```python
from build123d import *

# Parameters (mm, degrees)
PCB_START                  = -40
SK_PCB_W                   = 85
SK_PCB_H                   = 56
PCB_DEPTH                  = 1.6
BARRENOS_M2_5_START        = -40
SK_BARRENOS_M2_5_R         = 1.35
BARRENOS_M2_5_DEPTH        = 1.6
ETHERNET_START             = -38.4
SK_ETHERNET_W              = 21
SK_ETHERNET_H              = 16
ETHERNET_DEPTH             = 13.5
USB_START                  = -38.4
SK_USB_W                   = 17.5
SK_USB_H                   = 13
USB_DEPTH                  = 16
DISIPADOR_VENTILADOR_START = -38.4
SK_DISIPADOR_VENTILADOR_W  = 40
SK_DISIPADOR_VENTILADOR_H  = 38
DISIPADOR_VENTILADOR_DEPTH = 10


with BuildPart() as part:
    # Sk_PCB → PCB (new body)
    with BuildSketch(Plane.XY.offset(PCB_START)):
        with Locations((-52.5, 0)):
            Rectangle(SK_PCB_W, SK_PCB_H)
    extrude(amount=PCB_DEPTH)

    # Sk_Barrenos_M2-5 → Barrenos_M2-5 (cut)
    with BuildSketch(Plane.XY.offset(BARRENOS_M2_5_START)):
        with Locations((-13.5, -24.5)):
            Circle(SK_BARRENOS_M2_5_R)
        with Locations((-13.5, 24.5)):
            Circle(SK_BARRENOS_M2_5_R)
        with Locations((-71.5, -24.5)):
            Circle(SK_BARRENOS_M2_5_R)
        with Locations((-71.5, 24.5)):
            Circle(SK_BARRENOS_M2_5_R)
    extrude(amount=BARRENOS_M2_5_DEPTH, mode=Mode.SUBTRACT)

    # Sk_Ethernet → Ethernet (add)
    with BuildSketch(Plane.XY.offset(ETHERNET_START)):
        with Locations((-87.5, 16)):
            Rectangle(SK_ETHERNET_W, SK_ETHERNET_H)
    extrude(amount=ETHERNET_DEPTH)

    # Sk_USB → USB (add)
    with BuildSketch(Plane.XY.offset(USB_START)):
        with Locations((-89.25, -19.5)):
            Rectangle(SK_USB_W, SK_USB_H)
        with Locations((-89.25, -3.5)):
            Rectangle(SK_USB_W, SK_USB_H)
    extrude(amount=USB_DEPTH)

    # Sk_Disipador_ventilador → Disipador_ventilador (add)
    with BuildSketch(Plane.XY.offset(DISIPADOR_VENTILADOR_START)):
        with Locations((-42, -1)):
            Rectangle(SK_DISIPADOR_VENTILADOR_W, SK_DISIPADOR_VENTILADOR_H)
    extrude(amount=DISIPADOR_VENTILADOR_DEPTH)


solid = part.part
```
For this review, take the finished solid that the model builds, in its own axes (mm). A direction names the side the tool comes from. Coordinates: 2 decimals unless noted, no trailing zeros. Write each loop counter-clockwise with the first axis right and the second up, starting at its lowest first coordinate (ties: lowest second). Pieces come first, ordered by that corner, then holes. Notation, with made-up numbers: (83, 77.25) - (88, 77.25) arc R26 ccw to (88, 99.25) - close; hole circle Ø2 at (30.5, 25.25). An arc over 180 degrees is marked (long way). Put each result on its own line as item: value.
1. For pin 1 (10 mm diameter, centred on x = -45, y = 20, fed in from +Z); pin 2 (0.8 mm diameter, centred on y = 1.5, z = -39, fed in from -X); pin 3 (5 mm diameter, centred on y = 19.5, z = -35, fed in from +X); pin 4 (2.5 mm diameter, centred on x = -13.5, y = 24.5, fed in from -Z), all flat-tipped, find the tip position at first contact; note any pin that passes through.
Values found:
pin 1: z = -28.4
pin 2: x = -95
pin 3: x = -22
pin 4: through
2. Add section C-C, the plane z = -32.5. Give the boundary of the cut face in (x, y).
Values found:
outline: (-98, -26) - (-80.5, -26) - (-80.5, -13) - (-98, -13) - close; (-98, -10) - (-80.5, -10) - (-80.5, 3) - (-98, 3) - close; (-98, 8) - (-77, 8) - (-77, 24) - (-98, 24) - close; (-62, -20) - (-22, -20) - (-22, 18) - (-62, 18) - close
3. Add section B-B, the plane x = -13.5. Give the boundary of the cut face in (y, z), then the cut area to 3 significant figures.
Values found:
outline: (-28, -40) - (-25.85, -40) - (-25.85, -38.4) - (-28, -38.4) - close; (-23.15, -40) - (23.15, -40) - (23.15, -38.4) - (-23.15, -38.4) - close; (25.85, -40) - (28, -40) - (28, -38.4) - (25.85, -38.4) - close
area: 81.0 mm²
4. Add section D-D, the plane z = -23.75. Give the boundary of the cut face in (x, y), then the cut area to 3 significant figures.
Values found:
outline: (-98, -26) - (-80.5, -26) - (-80.5, -13) - (-98, -13) - close; (-98, -10) - (-80.5, -10) - (-80.5, 3) - (-98, 3) - close
area: 455 mm²
5. Wall thickness on probe 1 along Y at (x, z) = (-71.5, -39.2); probe 2 along X at (y, z) = (-3, -34.5); probe 3 along Y at (x, z) = (-93, -34.5): over which ranges is each line inside the solid? List them lowest first.
Values found:
probe 1: -28 to -25.85, -23.15 to 23.15, 25.85 to 28
probe 2: -98 to -80.5, -62 to -22
probe 3: -26 to -13, -10 to 3, 8 to 24
6. Add section A-A, the plane y = -24.5. Give the boundary of the cut face in (x, z), then the cut area to 3 significant figures.
Values found:
outline: (-98, -38.4) - (-95, -38.4) - (-95, -40) - (-72.85, -40) - (-72.85, -38.4) - (-80.5, -38.4) - (-80.5, -22.4) - (-98, -22.4) - close; (-70.15, -40) - (-14.85, -40) - (-14.85, -38.4) - (-70.15, -38.4) - close; (-12.15, -40) - (-10, -40) - (-10, -38.4) - (-12.15, -38.4) - close
area: 407 mm²
7. Machinability: for faces 5 (the flat face through (-97, -3, -38.4)), 6 (the flat face through (-88, 16, -24.9)), 7 (the flat face through (-42, 18, -33)), 8 (the flat face through (-42, -20, -33)), which of the approach directions +Z, -Z, +X, -X, +Y, -Y give a long, thin tool a straight path to every point of the face, cutting with its end or side? Answer none if there is none.
Values found:
face 5: -Z, -X, +Y, -Y
face 6: +Z, +X, -X, +Y
face 7: +Z, +X, +Y
face 8: +Z, +X, -Y
8. Mouldability with a two-part tool opening along X and no side actions: class faces 1 (the cylindrical face through (-70.253, 23.983, -39.211)), 2 (the flat face through (-88, 8, -32)), 3 (the flat face through (-77, 16, -32)), 4 (the flat face through (-10, 0, -39)) as released by +X, released by -X, zero draft, split by the parting line, or undercut.
Values found:
face 1: undercut
face 2: zero draft
face 3: undercut
face 4: released by +X
